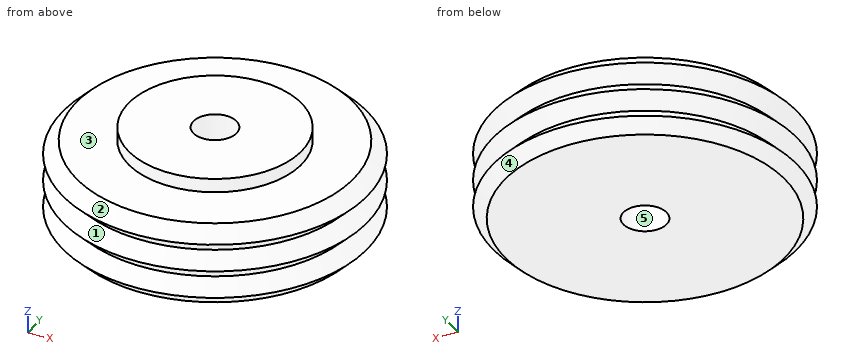
from build123d import *

# Parameters (mm, degrees)
SKETCH002_W   = 5
SKETCH002_H   = 4.7
ARRAY_Z_COUNT = 6
ARRAY_Z_PITCH = 1.6


with BuildPart() as obj1:
    # Sketch002 → Revolution002 (revolve)
    with BuildSketch(Plane.XZ):
        with Locations((7.5, 0.85)):
            Rectangle(SKETCH002_W, SKETCH002_H)
    revolve(axis=Axis((0, 0, 0), (0, 0, 1)))


with BuildPart() as innergroovetool:
    # Sketch001 → Revolution001 (revolve)
    with BuildSketch(Plane.XZ):
        Polygon((4, 3.2), (4, 1.6), (8, 1.6), (8.8, 2.4), (8, 3.2), align=None)
    revolve(axis=Axis((0, 0, 0), (0, 0, 1)))

    # Array Z: InnerGrooveTool ×6


with BuildPart() as innergroovetool_1:
    add(innergroovetool.part)
    with Locations(*[(0, 0, -i * ARRAY_Z_PITCH) for i in range(1, ARRAY_Z_COUNT)]):
        add(innergroovetool.part)

    # Common: intersect obj1
    add(obj1.part, mode=Mode.INTERSECT)


with BuildPart() as obj2:
    # Sketch → Revolution (revolve)
    with BuildSketch(Plane.XZ):
        Polygon((1.25, 4), (1.25, -1.5), (8, -1.5), (8, 3.2), (5, 3.2), (5, 4), align=None)
    revolve(axis=Axis((0, 0, 0), (0, 0, 1)))

    # Fusion001: union InnerGrooveTool
    add(innergroovetool_1.part)


solid = obj2.part
Verification items for the finished model (mm, model axes). Face numbers are marked on the shaded views. A direction names the side the tool comes from. Coordinates: 2 decimals unless noted, no trailing zeros. Loops run counter-clockwise (first coordinate to the right, second up) from the corner with the lowest first, then second, coordinate; pieces in that order, holes last. Notation, with made-up numbers: (82, -38.5) -> (141, -38.5) arc R21 ccw to (141, -26.5) -> close; hole circle Ø5 at (34.25, 19). An arc over 180 degrees is marked (long way). Answer as a JSON object with one key per item and string values. Group by question number.
Item 1: Sectioned sample at A-A on x = 0. Record the boundary of the cut face in (y, z), plus the area to 3 significant figures.
Item 2: Mould release check, pull along X, two halves, no side actions. Record for the marked faces 3, 4 and 5: +X half, -X half, draft (parallel to the pull), parting line (faces both ways), or undercut.
Item 3: Scan lines: probe 1 along X at (y, z) = (-1, 0.35); probe 2 along Z at (x, y) = (-4, 4.5); probe 3 along Y at (x, z) = (0, 0.2). Record each from-to range of solid material in increasing order.
Item 4: Depth check by flat-ended pin: pin 1 (3 mm diameter, centred on x = 0, y = 0, fed in from +Z); pin 2 (1.5 mm diameter, centred on y = -5.5, z = 1.5, fed in from -X); pin 3 (1 mm diameter, centred on x = 6.5, z = -0.5, fed in from -Y); pin 4 (2 mm diameter, centred on y = 3, z = -0.5, fed in from -X). Enter the tip coordinate at first touch or a pass-through.
Item 5: Tool access check on the marked faces 1 and 2. Record the directions out of +Z, -Z, +X, -X, +Y, -Y that give a thin tool (end or side, any length) a straight path to the whole face; none if there is none.
Item 6: Sectioned sample at C-C on z = 2.8. Record the boundary of the cut face in (x, y).
Evaluation:
{
 "1": {"outline": "(-8.8, -0.8) -> (-8.1, -1.5) -> (-1.25, -1.5) -> (-1.25, 4) -> (-5, 4) -> (-5, 3.2) -> (-8, 3.2) -> (-8.8, 2.4) -> (-8, 1.6) -> (-8.8, 0.8) -> (-8, 0) -> close; (1.25, -1.5) -> (8.1, -1.5) -> (8.8, -0.8) -> (8, 0) -> (8.8, 0.8) -> (8, 1.6) -> (8.8, 2.4) -> (8, 3.2) -> (5, 3.2) -> (5, 4) -> (1.25, 4) -> close", "area": "73.3 mm²"},
 "2": {"face 3": "draft", "face 4": "parting line", "face 5": "undercut"},
 "3": {"probe 1": "x = -8.29 to -0.75, 0.75 to 8.29", "probe 2": "z = -1.5 to 3.2", "probe 3": "y = -8.2 to -1.25, 1.25 to 8.2"},
 "4": {"pin 1": "stops at z = 4", "pin 2": "stops at x = -7.09", "pin 3": "stops at y = -6.34", "pin 4": "stops at x = -8.56"},
 "5": {"face 1": "none", "face 2": "+Z"},
 "6": {"outline": "circle Ø16.8 at (0, 0); hole circle Ø2.5 at (0, 0)"}
}
